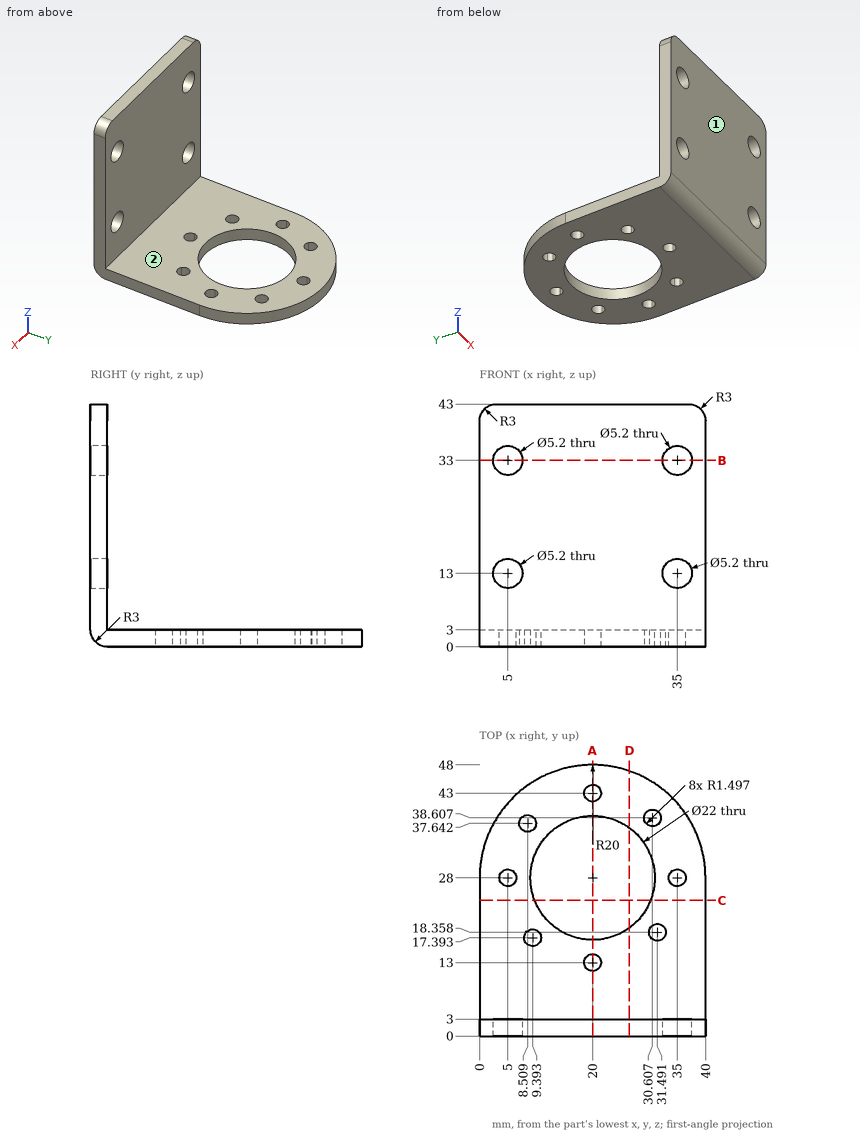
Part print with two shaded views. Sizes in mm from the minimum x, y, z corner. A direction names the side the tool comes from. Round coordinates to 2 decimals unless told otherwise and drop trailing zeros. Loops run counter-clockwise (first coordinate to the right, second up) from the corner with the lowest first, then second, coordinate; pieces in that order, holes last. Notation, with made-up numbers: (39, 33.25) - (66, 33.25) arc R22 cw to (66, 66.25) - close; hole circle Ø9 at (87.25, 65.25). An arc over 180 degrees is marked (long way). Answer as a JSON object with one key per item and string values.
Item 1: Band-saw the part on D-D on x = 26.5. List the corners of the cut face in (y, z) (1 decimal).
Output:
{"outline": "(0, 3) arc R3 ccw to (3, 0) - (19.1, 0) - (19.1, 3) - (3, 3) - (3, 43) - (0, 43) - close; (36.9, 0) - (46.9, 0) - (46.9, 3) - (36.9, 3) - close"}
Item 2: Wall check: L1, parallel to X at y = 28, z = 1.95; L2, parallel to X at y = 1, z = 33; L3, parallel to X at y = 2.5, z = 34. Give the ranges that are in metal, low to high.
Output:
{"L1": "0 to 3.5, 6.5 to 9, 31 to 33.5, 36.5 to 40", "L2": "0 to 2.4, 7.6 to 32.4, 37.6 to 40", "L3": "0 to 2.6, 7.4 to 32.6, 37.4 to 40"}
Item 3: Band-saw the part on B-B on z = 33. List the corners of the cut face in (x, y).
Output:
{"outline": "(0, 0) - (2.4, 0) - (2.4, 3) - (0, 3) - close; (7.6, 0) - (32.4, 0) - (32.4, 3) - (7.6, 3) - close; (37.6, 0) - (40, 0) - (40, 3) - (37.6, 3) - close"}
Item 4: Tool access for the marked faces 1 and 2: list every direction of +Z, -Z, +X, -X, +Y, -Y with a clear straight run to the whole face (end or side of a thin tool).
Output:
{"face 1": "+Z, -Z, +X, -X, -Y", "face 2": "+Z, +X, -X, +Y"}
Item 5: Band-saw the part on A-A on x = 20. List the corners of the cut face in (y, z), plus the area to 3 significant figures.
Output:
{"outline": "(0, 3) arc R3 ccw to (3, 0) - (11.5, 0) - (11.5, 3) - (3, 3) - (3, 43) - (0, 43) - close; (14.5, 0) - (17, 0) - (17, 3) - (14.5, 3) - close; (39, 0) - (41.5, 0) - (41.5, 3) - (39, 3) - close; (44.5, 0) - (48, 0) - (48, 3) - (44.5, 3) - close", "area": "178 mm2"}
Item 6: Pin check, flat tips, straight feed: pin 1 (4 mm diameter, centred on x = 17.5, y = 9, fed in from +Z); pin 2 (4 mm diameter, centred on x = 35, z = 33, fed in from -Y); pin 3 (7 mm diameter, centred on x = 5, z = 33, fed in from +Y). Stop position of each tip, or through.
Output:
{"pin 1": "z = 3", "pin 2": "through", "pin 3": "y = 3"}
Item 7: Band-saw the part on C-C on y = 24. List the corners of the cut face in (x, z).
Output:
{"outline": "(0, 0) - (9.75, 0) - (9.75, 3) - (0, 3) - close; (30.25, 0) - (40, 0) - (40, 3) - (30.25, 3) - close"}
